Can you work these out from the drawing? Everything is in mm from the part's minimum corner. A direction names the side the tool comes from. Give positions to 0.01 mm unless a question says otherwise; leave off trailing zeros. Order: outer loops, then holes, each group sorted by start corner. A loop starts at its lowest first (then second) coordinate and runs counter-clockwise, first axis right, second up. Notation, with made-up numbers: (74.5, 30) -> (121.5, 30) arc R17 ccw to (121.5, 62) -> close; hole circle Ø2 at (-9.75, -5). An arc over 180 degrees is marked (long way). Answer as CSV lines item,"result". Start each with the question number.
(1) I want a section at B-B (y = 46.5). Please give me the cut outline in (x, z), plus the area to 4 significant figures.
(2) I want a section at D-D (y = 31). Please give me the cut outline in (x, z), plus the area to 3 significant figures.
(3) I want a section at A-A (x = 5.75). Please give me the cut outline in (y, z), plus the area to 3 significant figures.
(4) We'd pull the mould along Y, two halves only. Please class the marked faces 4, 5, 6 and 7: released by +Y, released by -Y, zero draft, split by the parting line, or undercut.
(5) I want a section at C-C (z = 7.5). Please give me the cut outline in (x, y).
(6) Will this pin go through, and if not, where does the flat tip stop? pin 1 Ø2.5 at (y, z) = (21.5, 3) entering from +X.
(7) I need wall thicknesses on L1, parallel to Y at x = 7.75, z = 7.5; L2, parallel to Y at x = 8.5, z = 13; L3, parallel to X at y = 18.5, z = 11. Which ranges of each line are inside material? Lowest first, please.
(8) On a 3-axis mill with a long thin cutter (end or side, diameter ignored), from which of +Z, -Z, +X, -X, +Y, -Y can I reach the whole of each face in a straight line? I mean the marked faces 1, 2 and 3. Say none if no direction works.
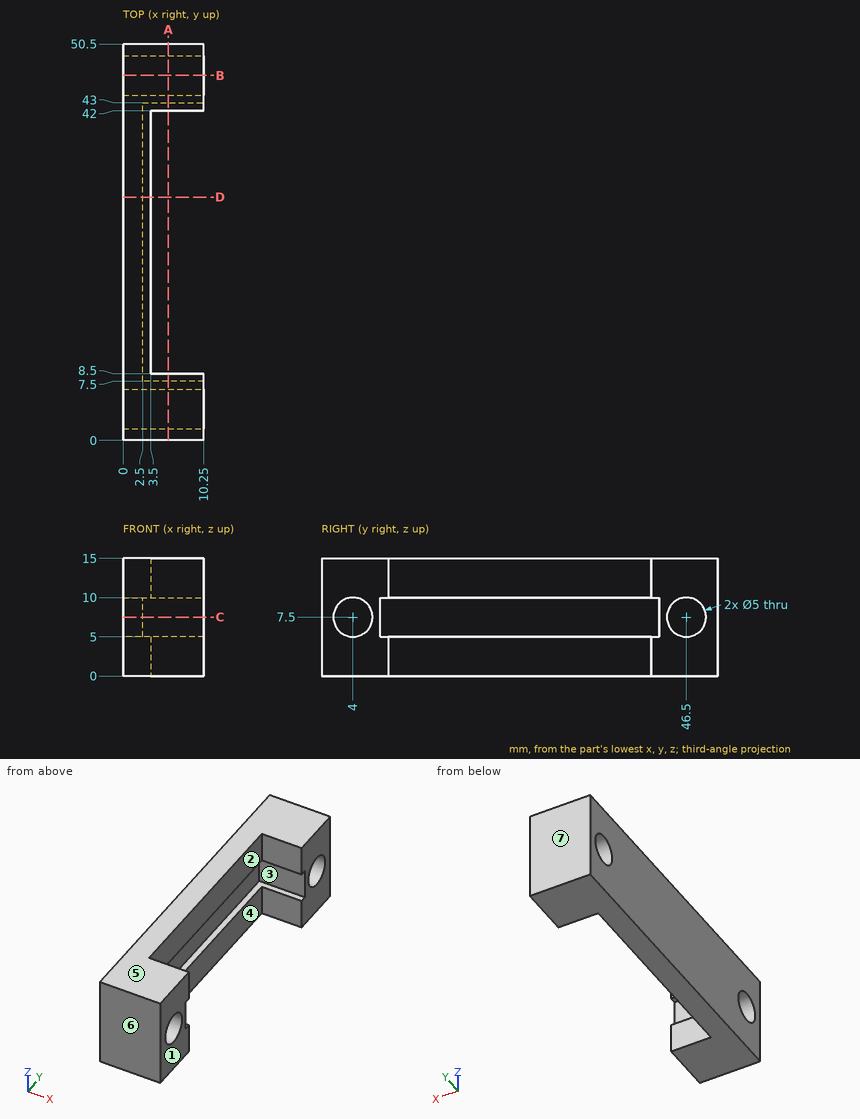
Final values:
1,outline,"(0, 0) -> (10.25, 0) -> (10.25, 5) -> (0, 5) -> close; (0, 10) -> (10.25, 10) -> (10.25, 15) -> (0, 15) -> close"
1,area,"102.5 mm²"
2,outline,"(0, 0) -> (3.5, 0) -> (3.5, 5) -> (2.5, 5) -> (2.5, 10) -> (3.5, 10) -> (3.5, 15) -> (0, 15) -> close"
2,area,"47.5 mm²"
3,outline,"(0, 0) -> (8.5, 0) -> (8.5, 5) -> (7.5, 5) -> (7.5, 10) -> (8.5, 10) -> (8.5, 15) -> (0, 15) -> close; (42, 0) -> (50.5, 0) -> (50.5, 15) -> (42, 15) -> (42, 10) -> (43, 10) -> (43, 5) -> (42, 5) -> close; hole circle Ø5 at (4, 7.5); hole circle Ø5 at (46.5, 7.5)"
3,area,"206 mm²"
4,face 4,"undercut"
4,face 5,"zero draft"
4,face 6,"released by -Y"
4,face 7,"released by +Y"
5,outline,"(0, 0) -> (10.25, 0) -> (10.25, 1.5) -> (0, 1.5) -> close; (0, 6.5) -> (10.25, 6.5) -> (10.25, 7.5) -> (2.5, 7.5) -> (2.5, 43) -> (10.25, 43) -> (10.25, 44) -> (0, 44) -> close; (0, 49) -> (10.25, 49) -> (10.25, 50.5) -> (0, 50.5) -> close"
6,pin 1,"x = 3.5"
7,L1,"0 to 1.5, 6.5 to 7.5, 43 to 44, 49 to 50.5"
7,L2,"0 to 8.5, 42 to 50.5"
7,L3,"0 to 3.5"
8,face 1,"+Z, -Z, +X, +Y, -Y"
8,face 2,"+Z, -Z, +X"
8,face 3,"+X"
